```python
from build123d import *

# Parameters (mm, degrees)
F0_W     = 10.73
F0_H     = 5.24
F1_DEPTH = 11.08
F3_D     = 3.9
F3_DEPTH = 12
F5_D     = 5.5


with BuildPart() as f1:
    # F0 (on Top) → F1 (new body)
    with BuildSketch(Plane.XY):
        Polygon((0, 6.275), (-15.84, 6.275), (-15.84, -6.275), (0, -6.275), (0, -2.62), (0, 2.62), align=None)
        with BuildLine():
            Line((-12.84, -3.11), (-12.84, 3.11))
            Line((-12.84, 3.11), (-9.62, 3.11))
            Line((-9.62, 3.11), (-9.62, 2.2))
            Line((-9.62, 2.2), (-4.82, 2.2))
            ThreePointArc((-4.82, 2.2), (-3.264365, 1.555635), (-2.62, 0))
            ThreePointArc((-2.62, 0), (-3.264365, -1.555635), (-4.82, -2.2))
            Line((-4.82, -2.2), (-9.62, -2.2))
            Line((-9.62, -2.2), (-9.62, -3.11))
            Line((-9.62, -3.11), (-12.84, -3.11))
        make_face(mode=Mode.SUBTRACT)
        with Locations((5.365, 0)):
            Rectangle(F0_W, F0_H)
    extrude(amount=F1_DEPTH)

    # F3
    with Locations(Plane(origin=(-15.84, 0, 0), x_dir=(0, -1, 0), z_dir=(-1, 0, 0))):
        with Locations((0, 5.54)):
            Hole(F3_D / 2, depth=F3_DEPTH)

    # F5 (through all)
    with Locations(Plane.XZ.offset(2.62)):
        with Locations((5.365, 5.54)):
            Hole(F5_D / 2)


solid = f1.part
```
CAD build for the part. Positions are in the model's coordinates, mm. A direction names the side the tool comes from. Round coordinates to 2 decimals unless told otherwise and drop trailing zeros. Write each loop counter-clockwise with the first axis right and the second up, starting at its lowest first coordinate (ties: lowest second). Pieces come first, ordered by that corner, then holes.
Item 1: Mould opens along Z. For faces 5 (the flat face through (-2.7, 1.5, 0)), 6 (the flat face through (3, 2.62, 3)), 7 (the flat face through (-2.7, 1.5, 11.08)), 8 (the cylindrical face through (3.89, 0.04, 7.86)) say: released by +Z, released by -Z, zero draft, split by the parting line, or undercut.
Filled in:
face 5: released by -Z
face 6: zero draft
face 7: released by +Z
face 8: undercut
Item 2: Band-saw the part on A-A on x = -12.25. Write the cut outline in (y, z) (3 decimals).
Filled in:
outline: (-6.275, 0) - (-3.11, 0) - (-3.11, 11.08) - (-6.275, 11.08) - close; (3.11, 0) - (6.275, 0) - (6.275, 11.08) - (3.11, 11.08) - close
Item 3: Band-saw the part on B-B on z = 5.54. Write the cut outline in (x, y) (3 decimals), then the cut area to 3 significant figures.
Filled in:
outline: (-15.84, -6.275) - (0, -6.275) - (0, -2.62) - (2.615, -2.62) - (2.615, 2.62) - (0, 2.62) - (0, 6.275) - (-15.84, 6.275) - (-15.84, 1.95) - (-12.84, 1.95) - (-12.84, 3.11) - (-9.62, 3.11) - (-9.62, 2.2) - (-4.82, 2.2) arc R2.2 cw to (-4.82, -2.2) - (-9.62, -2.2) - (-9.62, -3.11) - (-12.84, -3.11) - (-12.84, -1.95) - (-15.84, -1.95) - close; (8.115, -2.62) - (10.73, -2.62) - (10.73, 2.62) - (8.115, 2.62) - close
area: 166 mm2
Item 4: Band-saw the part on D-D on y = 4.75. Write the cut outline in (x, z), then the cut area to 3 significant figures.
Filled in:
outline: (-15.84, 0) - (0, 0) - (0, 11.08) - (-15.84, 11.08) - close
area: 176 mm2
Item 5: Drill centre lines: L1, parallel to Z at x = -14.3, y = 0; L2, parallel to X at y = 2.75, z = 3; L3, parallel to Y at x = -9, z = 9 (3 decimals). Where is each one in solid material? Low to high.
Filled in:
L1: z = 0 to 3.59, 7.49 to 11.08
L2: x = -15.84 to -12.84, -9.62 to 0
L3: y = -6.275 to -2.2, 2.2 to 6.275
Item 6: Tool access for faces 1 (the cylindrical face through (-14.319, -1.547, 4.353)), 2 (the flat face through (3, -2.62, 3)), 3 (the flat face through (-9.62, -2.6, 5.5)), 4 (the flat face through (-15.84, 0, 3)): list every direction of +Z, -Z, +X, -X, +Y, -Y with a clear straight run to the whole face (end or side of a thin tool).
Filled in:
face 1: -X
face 2: +Z, -Z, +X, -Y
face 3: +Z, -Z
face 4: +Z, -Z, -X, +Y, -Y
Item 7: Band-saw the part on C-C on z = 2.5. Write the cut outline in (x, y) (3 decimals), then the cut area to 3 significant figures.
Filled in:
outline: (-15.84, -6.275) - (0, -6.275) - (0, -2.62) - (10.73, -2.62) - (10.73, 2.62) - (0, 2.62) - (0, 6.275) - (-15.84, 6.275) - close; hole (-12.84, -3.11) - (-9.62, -3.11) - (-9.62, -2.2) - (-4.82, -2.2) arc R2.2 ccw to (-4.82, 2.2) - (-9.62, 2.2) - (-9.62, 3.11) - (-12.84, 3.11) - close
area: 206 mm2
Item 8: Drop flat-ended pins along their axis: pin 1 Ø2 at (x, z) = (1.5, 1.5) entering from +Y; pin 2 Ø1.8 at (y, z) = (4.5, 4.5) entering from +X; pin 3 Ø3 at (y, z) = (0, 5.54) entering from -X. Give the stop position or say it passes through.
Filled in:
pin 1: stops at y = 2.62
pin 2: stops at x = 0
pin 3: stops at x = -3.21
